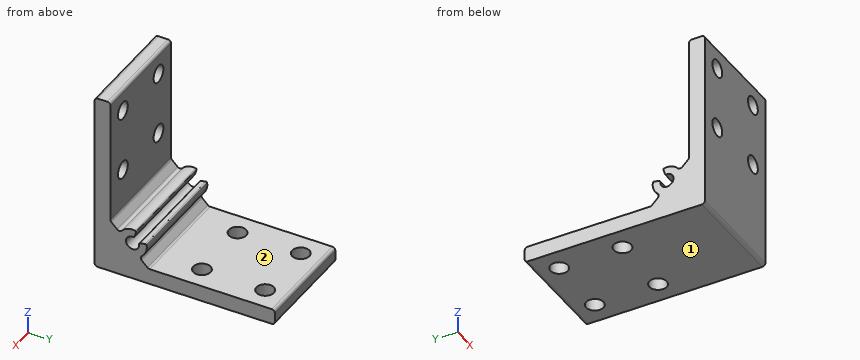
from build123d import *

# Parameters (mm, degrees)
BOSS_EXTRUDE1_DEPTH      = 17
BOSS_EXTRUDE1_DEPTH_BACK = 17
SKETCH2_R                = 2.75
CUT_EXTRUDE1_DEPTH       = 5
SKETCH3_R                = 2.75
CUT_EXTRUDE2_DEPTH       = 5
SKETCH4_R                = 2.75
CUT_EXTRUDE3_DEPTH       = 5
SKETCH5_R                = 2.75
CUT_EXTRUDE4_DEPTH       = 5
SKETCH6_R                = 2.75
CUT_EXTRUDE5_DEPTH       = 5
SKETCH7_R                = 2.75
CUT_EXTRUDE6_DEPTH       = 5
SKETCH8_R                = 2.75
CUT_EXTRUDE7_DEPTH       = 5
SKETCH9_R                = 2.75
CUT_EXTRUDE8_DEPTH       = 5


with BuildPart() as part:
    # Sketch1 → Boss-Extrude1 (new, two sides: drawn at the far end of the back side and taken through both)
    with BuildSketch(Plane(origin=(0, 0, 0), x_dir=(0, 0, -1), z_dir=(1, 0, 0)).offset(-BOSS_EXTRUDE1_DEPTH_BACK)):
        with BuildLine():
            Line((-56, 0), (-1, 0))
            ThreePointArc((-1, 0), (-0.292893219, 0.292893219), (0, 1))
            Line((0, 1), (0, 56))
            ThreePointArc((0, 56), (-0.292893219, 56.707106781), (-1, 57))
            Line((-1, 57), (-4, 57))
            ThreePointArc((-4, 57), (-4.707106781, 56.707106781), (-5, 56))
            Line((-5, 56), (-5, 17.414213562))
            ThreePointArc((-5, 17.414213562), (-5.076120467, 17.03153013), (-5.292893219, 16.707106781))
            Line((-5.292893219, 16.707106781), (-7.121957509, 14.878042491))
            ThreePointArc((-7.121957509, 14.878042491), (-7.866746832, 14.585859511), (-8.587416237, 14.93330395))
            ThreePointArc((-8.587416237, 14.93330395), (-10.519537564, 16.249497732), (-12.851234525, 16.418755456))
            ThreePointArc((-12.851234525, 16.418755456), (-13.048766707, 16.283360738), (-13.084263382, 16.046526031))
            Line((-13.084263382, 16.046526031), (-12.616293745, 14.300039569))
            ThreePointArc((-12.616293745, 14.300039569), (-12.492491512, 14.127781044), (-12.285701536, 14.080474617))
            ThreePointArc((-12.285701536, 14.080474617), (-10.515075746, 10.515075773), (-14.080474622, 12.285701498))
            ThreePointArc((-14.080474622, 12.285701498), (-14.127781033, 12.492491496), (-14.300039569, 12.616293745))
            Line((-14.300039569, 12.616293745), (-16.046526031, 13.084263382))
            ThreePointArc((-16.046526031, 13.084263382), (-16.283360688, 13.048766739), (-16.418755434, 12.851234641))
            ThreePointArc((-16.418755434, 12.851234641), (-16.249497766, 10.51953766), (-14.933304014, 8.587416292))
            ThreePointArc((-14.933304014, 8.587416292), (-14.585859513, 7.866746874), (-14.878042491, 7.121957509))
            Line((-14.878042491, 7.121957509), (-16.707106781, 5.292893219))
            ThreePointArc((-16.707106781, 5.292893219), (-17.03153013, 5.076120467), (-17.414213562, 5))
            Line((-17.414213562, 5), (-56, 5))
            ThreePointArc((-56, 5), (-56.707106781, 4.707106781), (-57, 4))
            Line((-57, 4), (-57, 1))
            ThreePointArc((-57, 1), (-56.707106781, 0.292893219), (-56, 0))
        make_face()
    extrude(amount=BOSS_EXTRUDE1_DEPTH + BOSS_EXTRUDE1_DEPTH_BACK)

    # Sketch2 → Cut-Extrude1 (cut)
    with BuildSketch(Plane(origin=(0, 0, 0), x_dir=(1, 0, 0), z_dir=(0, 1, 0))):
        with Locations(Location((-10, -30, 0), (0, 0, 270))):
            Circle(SKETCH2_R)
    extrude(amount=CUT_EXTRUDE1_DEPTH, mode=Mode.SUBTRACT)

    # Sketch3 → Cut-Extrude2 (cut)
    with BuildSketch(Plane(origin=(0, 0, 0), x_dir=(1, 0, 0), z_dir=(0, 1, 0))):
        with Locations(Location((-10, -50, 0), (0, 0, 270))):
            Circle(SKETCH3_R)
    extrude(amount=CUT_EXTRUDE2_DEPTH, mode=Mode.SUBTRACT)

    # Sketch4 → Cut-Extrude3 (cut)
    with BuildSketch(Plane(origin=(0, 0, 0), x_dir=(1, 0, 0), z_dir=(0, 1, 0))):
        with Locations(Location((10, -30, 0), (0, 0, 270))):
            Circle(SKETCH4_R)
    extrude(amount=CUT_EXTRUDE3_DEPTH, mode=Mode.SUBTRACT)

    # Sketch5 → Cut-Extrude4 (cut)
    with BuildSketch(Plane(origin=(0, 0, 0), x_dir=(1, 0, 0), z_dir=(0, 1, 0))):
        with Locations(Location((10, -50, 0), (0, 0, 270))):
            Circle(SKETCH5_R)
    extrude(amount=CUT_EXTRUDE4_DEPTH, mode=Mode.SUBTRACT)

    # Sketch6 → Cut-Extrude5 (cut)
    with BuildSketch(Plane.XY):
        with Locations((-10, 30)):
            Circle(SKETCH6_R)
    extrude(amount=CUT_EXTRUDE5_DEPTH, mode=Mode.SUBTRACT)

    # Sketch7 → Cut-Extrude6 (cut)
    with BuildSketch(Plane.XY):
        with Locations((10, 30)):
            Circle(SKETCH7_R)
    extrude(amount=CUT_EXTRUDE6_DEPTH, mode=Mode.SUBTRACT)

    # Sketch8 → Cut-Extrude7 (cut)
    with BuildSketch(Plane.XY):
        with Locations((-10, 50)):
            Circle(SKETCH8_R)
    extrude(amount=CUT_EXTRUDE7_DEPTH, mode=Mode.SUBTRACT)

    # Sketch9 → Cut-Extrude8 (cut)
    with BuildSketch(Plane.XY):
        with Locations((10, 50)):
            Circle(SKETCH9_R)
    extrude(amount=CUT_EXTRUDE8_DEPTH, mode=Mode.SUBTRACT)


solid = part.part
Could you check a few things on this model? Use its own coordinates, in mm. Face numbers are marked on the shaded views. A direction names the side the tool comes from. Coordinates: 2 decimals unless noted, no trailing zeros. Order: outer loops, then holes, each group sorted by start corner. A loop starts at its lowest first (then second) coordinate and runs counter-clockwise, first axis right, second up. Notation, with made-up numbers: (81, -33) -> (111, -33) arc R13 ccw to (111, -15) -> close; hole circle Ø10 at (87, 40.25). An arc over 180 degrees is marked (long way). One line per question, with ' | ' between items.
Q1. Imagine slicing it at D-D on y = 11. Please give me the cut outline in (x, z), and give its area (3 significant figures).
Return value:
outline: (-17, 0) -> (17, 0) -> (17, 10.15) -> (-17, 10.15) -> close; (-17, 13.85) -> (17, 13.85) -> (17, 16.39) -> (-17, 16.39) -> close | area: 432 mm²
Q2. I'm going to push flat-ended pins straight in: P1, Ø6.5, axis at x = -10, z = 50, coming from the +Y side; P2, Ø10, axis at x = -4.5, y = 31, coming from the +Z side. Where does each tip first touch, or does it pass through?
Return value:
P1: y = 5 | P2: z = 5
Q3. Imagine slicing it at C-C on x = 3. Please give me the cut outline in (y, z), and give its area (3 significant figures).
Return value:
outline: (0, 1) arc R1 ccw to (1, 0) -> (56, 0) arc R1 ccw to (57, 1) -> (57, 4) arc R1 ccw to (56, 5) -> (17.41, 5) arc R1 cw to (16.71, 5.29) -> (14.88, 7.12) arc R1 cw to (14.93, 8.59) arc R4.5 ccw to (16.42, 12.85) arc R0.3 ccw to (16.05, 13.08) -> (14.3, 12.62) arc R0.3 ccw to (14.08, 12.29) arc R2.1 cw (long way) to (12.29, 14.08) arc R0.3 ccw to (12.62, 14.3) -> (13.08, 16.05) arc R0.3 ccw to (12.85, 16.42) arc R4.5 ccw to (8.59, 14.93) arc R1 cw to (7.12, 14.88) -> (5.29, 16.71) arc R1 cw to (5, 17.41) -> (5, 56) arc R1 ccw to (4, 57) -> (1, 57) arc R1 ccw to (0, 56) -> close | area: 639 mm²
Q4. Imagine slicing it at A-A on z = 30. Please give me the cut outline in (x, y).
Return value:
outline: (-17, 0) -> (-12.75, 0) -> (-12.75, 5) -> (-17, 5) -> close; (-7.25, 0) -> (7.25, 0) -> (7.25, 5) -> (-7.25, 5) -> close; (12.75, 0) -> (17, 0) -> (17, 5) -> (12.75, 5) -> close
Q5. If I drill on L1, parallel to X at y = 1.45, z = 30; L2, parallel to Y at x = 10, z = 2; L3, parallel to X at y = 3, z = 29, over which ranges is the centre line in solid material (lowest first)?
Return value:
L1: -17 to -12.75, -7.25 to 7.25, 12.75 to 17 | L2: 0 to 27.25, 32.75 to 47.25, 52.75 to 57 | L3: -17 to -12.56, -7.44 to 7.44, 12.56 to 17
Q6. On a 3-axis mill with a long thin cutter (end or side, diameter ignored), from which of +Z, -Z, +X, -X, +Y, -Y can I reach the whole of each face in a straight line? I mean the marked faces 1 and 2. Say none if no direction works.
Return value:
face 1: -Z, +X, -X, +Y, -Y | face 2: +Z, +X, -X, +Y
